The listing builds one solid part. Answer for the finished solid, in the listing's coordinates (mm). A direction names the side the tool comes from. Give positions to 0.01 mm unless a question says otherwise; leave off trailing zeros. Loops run counter-clockwise (first coordinate to the right, second up) from the corner with the lowest first, then second, coordinate; pieces in that order, holes last. Notation, with made-up numbers: (-20, 33) - (-8, 33) arc R30 cw to (-8, 72) - close; hole circle Ø1 at (-30.75, 70.5). An arc over 180 degrees is marked (long way). Answer as CSV lines item,"result". Start each with the question number.
1) A cutting plane is placed at D-D (x = 12). Determine the outline of the cut face in (y, z).
2) Find the intervals of material crossed by line 1 along Z through (x, y) = (9.25, 0.8); line 2 along X through (y, z) = (0.55, -5); line 3 along Y through (x, z) = (2.5, -10.75), in increasing order.
3) A cutting plane is placed at C-C (x = 2.25). Determine the outline of the cut face in (y, z), and give its area (3 significant figures).
4) A cutting plane is placed at B-B (z = -23.25). Determine the outline of the cut face in (x, y), and give its area (3 significant figures).
5) A cutting plane is placed at A-A (y = 6). Determine the outline of the cut face in (x, z).
6) For a pull along Z with two mould halves and no side action, classify faces 4 (the face through (0, 4, -13)), 5 (the face through (17.19, 5.09, -4.94)), 6 (the face through (9.17, 2.41, -20.54)), 7 (the face through (9, 2, -25.41)) as pulls with the +Z half, pulls with the -Z half, needs draft (parallel to the pull), parting line crosses it, or undercut.
7) For faces 1 (the face through (9.06, 1, -4.13)), 2 (the face through (2, 7.5, -13)), 3 (the face through (17.755, 7.243, -4.459)), determine the directions among +Z, -Z, +X, -X, +Y, -Y from which every point of the face is accessible in a straight line to the end or side of a thin tool.
8) Flat-ended cylindrical pins translate along their axes: pin 1 (3 mm diameter, centred on x = 9.25, z = -5, fed in from +Y); pin 2 (3.5 mm diameter, centred on x = 1, z = -12.5, fed in from +Y); pin 3 (1.1 mm diameter, centred on x = 17.05, z = -5, fed in from -Y); pin 4 (8 mm diameter, centred on x = 11, z = -4, fed in from +Y). Find the tip coordinate at first contact, or state that the pin passes through.
```python
from build123d import *

# Parameters (mm, degrees)
SKETCH2_W                 = 18.5
SKETCH2_H                 = 25.41
BOSS_EXTRUDE1_DEPTH       = 9
CUT_EXTRUDE1_DEPTH        = 25.41
F_2_56_TAPPED_HOLE1_D     = 1.778
F_2_56_TAPPED_HOLE1_DEPTH = 1.96583491
F_2_56_TAPPED_HOLE1_TIP   = 0.53416509
F_2_56_TAPPED_HOLE2_D     = 1.778
F_2_56_TAPPED_HOLE2_DEPTH = 3.46583491
F_2_56_TAPPED_HOLE2_TIP   = 0.53416509
CUT_EXTRUDE3_DEPTH        = 33.694312961
CUT_EXTRUDE3_DEPTH_BACK   = 25.41


with BuildPart() as part:
    # Sketch2 → Boss-Extrude1 (new body)
    with BuildSketch(Plane(origin=(0, 0, 0), x_dir=(1, 0, 0), z_dir=(0, 1, 0))):
        with Locations((9.25, 12.705)):
            Rectangle(SKETCH2_W, SKETCH2_H)
    extrude(amount=BOSS_EXTRUDE1_DEPTH)

    # Sketch6 → Cut-Extrude1 (cut)
    with BuildSketch(Plane.XY):
        with BuildLine():
            Line((2.9, 9), (15.6, 9))
            ThreePointArc((15.6, 9), (9.25, 2.65), (2.9, 9))
        make_face()
    extrude(amount=-CUT_EXTRUDE1_DEPTH, mode=Mode.SUBTRACT)

    # #2-56 Tapped Hole1
    with Locations(Plane(origin=(0, 0, 0), x_dir=(-1, 0, 0), z_dir=(0, -1, 0))):
        with Locations((-9.25, 20.41), (-9.25, 5)):
            Hole(F_2_56_TAPPED_HOLE1_D / 2, depth=F_2_56_TAPPED_HOLE1_DEPTH)
            with Locations((0, 0, -(F_2_56_TAPPED_HOLE1_DEPTH + F_2_56_TAPPED_HOLE1_TIP / 2))):  # 118° drill point
                Cone(0, F_2_56_TAPPED_HOLE1_D / 2, F_2_56_TAPPED_HOLE1_TIP, mode=Mode.SUBTRACT)

    # #2-56 Tapped Hole2
    with Locations(Plane(origin=(0, 9, 0), x_dir=(1, 0, 0), z_dir=(0, 1, 0))):
        with Locations((17.05, 20.41), (17.05, 5)):
            Hole(F_2_56_TAPPED_HOLE2_D / 2, depth=F_2_56_TAPPED_HOLE2_DEPTH)
            with Locations((0, 0, -(F_2_56_TAPPED_HOLE2_DEPTH + F_2_56_TAPPED_HOLE2_TIP / 2))):  # 118° drill point
                Cone(0, F_2_56_TAPPED_HOLE2_D / 2, F_2_56_TAPPED_HOLE2_TIP, mode=Mode.SUBTRACT)

    # Sketch14 → Cut-Extrude3 (cut, two sides: drawn at the far end of the back side and taken through both)
    with BuildSketch(Plane(origin=(0, 0, -25.41), x_dir=(-1, 0, 0), z_dir=(0, 0, -1)).offset(-CUT_EXTRUDE3_DEPTH_BACK)):
        Polygon((0, 60.146081223), (0, 9), (0, 7.5), (-3.246658661, 7.5), (-2.9, 9), (8.616604878, 58.832614185), (24.031387378, 159.956651774), (15.4147825, 161.270118812), align=None)
    extrude(amount=CUT_EXTRUDE3_DEPTH + CUT_EXTRUDE3_DEPTH_BACK, mode=Mode.SUBTRACT)


with BuildPart() as cut_extrude3_kept_piece:
    # of the separate pieces the step leaves, the one the design keeps (cut_extrude3_pieces_kept)
    add(part.part.solids().sort_by_distance((0, 0, 0))[0])


solid = cut_extrude3_kept_piece.part
```
Ans:
1,outline,"(0, -25.41) - (3.28, -25.41) - (3.28, 0) - (0, 0) - close"
2,line 1,"-25.41 to -21.3, -19.52 to -5.89, -4.11 to 0"
2,line 2,"0 to 8.36, 10.14 to 18.5"
2,line 3,"0 to 7.5"
3,outline,"(0, -25.41) - (7.5, -25.41) - (7.5, 0) - (0, 0) - close"
3,area,"191 mm2"
4,outline,"(0, 0) - (18.5, 0) - (18.5, 9) - (15.6, 9) arc R6.35 cw to (3.08, 7.5) - (0, 7.5) - close"
4,area,"98.7 mm2"
5,outline,"(0, -25.41) - (3.65, -25.41) - (3.65, 0) - (0, 0) - close; (14.85, -25.41) - (18.5, -25.41) - (18.5, 0) - (14.85, 0) - close; hole circle Ø1.78 at (17.05, -20.41); hole circle Ø1.78 at (17.05, -5)"
6,face 4,"needs draft"
6,face 5,"undercut"
6,face 6,"undercut"
6,face 7,"pulls with the -Z half"
7,face 1,"-Y"
7,face 2,"+Z, -Z, -X, +Y"
7,face 3,"+Y"
8,pin 1,"y = 2.83"
8,pin 2,"y = 7.5"
8,pin 3,"y = 0"
8,pin 4,"y = 6.31"
